Input: part model. Units: mm. Frame: model coordinates. A direction names the side the tool comes from. Round coordinates to 2 decimals unless told otherwise and drop trailing zeros. Loops run counter-clockwise (first coordinate to the right, second up) from the corner with the lowest first, then second, coordinate; pieces in that order, holes last. Notation, with made-up numbers: M 35.5,-40 L 57.5,-40 A22 cw 57.5,-2 Z; hole C -0.75,18.25 d2. An arc over 180 degrees is marked long. Return JSON: item names as keys, results as strings. Group by question number.
1) Contact query for flat-ended pins moving along their axis: P1, Ø1.2, axis at x = -194.5, z = 1.5, coming from the +Y side; P2, Ø1.5, axis at y = 70.5, z = 0.5, coming from the -X side. Output: stop coordinate, or through.
2) Mould query, pull axis X, two halves, no side actions, for faces 3 (the face through (-199.298, 76, 1)), 4 (the face through (-157, 69.019, 1)), 5 (the face through (-119.098, 79, 1)), 6 (the face through (-113.953, 82.117, 1.234)). Classes: +X half, -X half, draft (parallel to the pull), parting line (faces both ways), or undercut.
3) Access query for faces 1 (the face through (-113.098, 76, 1)), 2 (the face through (-118, 76.019, 1)). Directions: +Z, -Z, +X, -X, +Y, -Y. A direction counts if a zero-diameter tool reaches every point of the face in a straight line with its end or side. Return the directions, or none.
4) Section B-B (z = 0.95). Output: boundary loops of the cut face in (x, y), plus the area to 3 significant figures.
5) Material intervals for line 1 (X direction, y = 78.75, z = 0.55); line 2 (X direction, y = 72.25, z = 0.2); line 3 (X direction, y = 70.75, z = 1.6), sorted ascending. Write a range as from..to.
6) Section A-A (y = 78.5). Output: boundary loops of the cut face in (x, z).
from build123d import *

# Parameters (mm, degrees)
RESSALTO_EXTRUS_O1_DEPTH = 2.5
FILETE1_R                = 0.1


with BuildPart() as part:
    # Esboço1 → Ressalto-extrusão1 (new body)
    with BuildSketch(Plane.XY):
        with BuildLine():
            ThreePointArc((-199.297641475, 72.518779678), (-198.272493356, 70.044033295), (-195.797641475, 69.019139891))
            Line((-195.797641475, 69.019139891), (-116.597641475, 69.019139891))
            ThreePointArc((-116.597641475, 69.019139891), (-114.122789593, 70.044033295), (-113.097641475, 72.518779678))
            Line((-113.097641475, 72.518779678), (-113.097641475, 80.019139873))
            ThreePointArc((-113.097641475, 80.019139873), (-113.976321131, 82.140460216), (-116.097641475, 83.019139873))
            Line((-116.097641475, 83.019139873), (-116.597641475, 83.019139873))
            Line((-116.597641475, 83.019139873), (-116.597641475, 76.019139873))
            Line((-116.597641475, 76.019139873), (-119.097641475, 76.019139873))
            Line((-119.097641475, 76.019139873), (-119.097641475, 83.019139873))
            Line((-119.097641475, 83.019139873), (-135.097641475, 83.019139873))
            Line((-135.097641475, 83.019139873), (-141.097641475, 83.019139873))
            Line((-141.097641475, 83.019139873), (-171.297641475, 83.019139873))
            Line((-171.297641475, 83.019139873), (-177.297641475, 83.019139873))
            Line((-177.297641475, 83.019139873), (-193.297641475, 83.019139873))
            Line((-193.297641475, 83.019139873), (-193.297641475, 76.019139873))
            Line((-193.297641475, 76.019139873), (-195.797641475, 76.019139873))
            Line((-195.797641475, 76.019139873), (-195.797641475, 83.019139873))
            Line((-195.797641475, 83.019139873), (-196.297641475, 83.019139873))
            ThreePointArc((-196.297641475, 83.019139873), (-198.418961818, 82.140460216), (-199.297641475, 80.019139873))
            Line((-199.297641475, 80.019139873), (-199.297641475, 72.518779678))
        make_face()
    extrude(amount=RESSALTO_EXTRUS_O1_DEPTH)

    # Filete1
    filete1_edges = [part.edges().sort_by_distance(p)[0] for p in [
        (-199.297641475, 76.268959775, 2.5),
        (-195.797641475, 79.519139873, 0),
        (-194.547641475, 76.019139873, 0),
        (-198.272493356, 70.044033295, 2.5),
        (-193.297641475, 79.519139873, 0),
        (-156.197641475, 83.019139873, 0),
        (-119.097641475, 79.519139873, 0),
        (-117.847641475, 76.019139873, 0),
        (-116.597641475, 79.519139873, 0),
        (-116.347641475, 83.019139873, 0),
        (-113.976321131, 82.140460216, 0),
        (-113.097641475, 76.268959775, 0),
        (-156.197641475, 69.019139891, 2.5),
        (-114.122789593, 70.044033295, 0),
        (-156.197641475, 69.019139891, 0),
        (-198.272493356, 70.044033295, 0),
        (-199.297641475, 76.268959775, 0),
        (-198.418961818, 82.140460216, 0),
        (-196.047641475, 83.019139873, 0),
        (-114.122789593, 70.044033295, 2.5),
        (-113.097641475, 76.268959775, 2.5),
        (-195.797641475, 83.019139873, 1.25),
        (-195.797641475, 76.019139873, 1.25),
        (-193.297641475, 76.019139873, 1.25),
        (-193.297641475, 83.019139873, 1.25),
        (-119.097641475, 83.019139873, 1.25),
        (-119.097641475, 76.019139873, 1.25),
        (-116.597641475, 76.019139873, 1.25),
        (-116.597641475, 83.019139873, 1.25),
        (-113.976321131, 82.140460216, 2.5),
        (-116.347641475, 83.019139873, 2.5),
        (-116.597641475, 79.519139873, 2.5),
        (-117.847641475, 76.019139873, 2.5),
        (-119.097641475, 79.519139873, 2.5),
        (-196.047641475, 83.019139873, 2.5),
        (-156.197641475, 83.019139873, 2.5),
        (-193.297641475, 79.519139873, 2.5),
        (-194.547641475, 76.019139873, 2.5),
        (-195.797641475, 79.519139873, 2.5),
        (-198.418961818, 82.140460216, 2.5),
    ]]
    fillet(filete1_edges, radius=FILETE1_R)


solid = part.part
Returned:
{
 "1": {"P1": "stops at y = 76.02", "P2": "stops at x = -199.06"},
 "2": {"face 3": "-X half", "face 4": "draft", "face 5": "undercut", "face 6": "+X half"},
 "3": {"face 1": "+Z, -Z, +X, +Y, -Y", "face 2": "+Z, -Z, +Y"},
 "4": {"outline": "M -199.3,72.52 A3.5 ccw -195.8,69.02 L -116.6,69.02 A3.5 ccw -113.1,72.52 L -113.1,80.02 A3 ccw -116.1,83.02 L -116.5,83.02 A0.1 ccw -116.6,82.92 L -116.6,76.12 A0.1 cw -116.7,76.02 L -119,76.02 A0.1 cw -119.1,76.12 L -119.1,82.92 A0.1 ccw -119.2,83.02 L -193.2,83.02 A0.1 ccw -193.3,82.92 L -193.3,76.12 A0.1 cw -193.4,76.02 L -195.7,76.02 A0.1 cw -195.8,76.12 L -195.8,82.92 A0.1 ccw -195.9,83.02 L -196.3,83.02 A3 ccw -199.3,80.02 Z", "area": "1,160 mm^2"},
 "5": {"line 1": "x = -199.3..-195.8, -193.3..-119.1, -116.6..-113.1", "line 2": "x = -199.29..-113.11", "line 3": "x = -198.82..-113.58"},
 "6": {"outline": "M -199.3,0.1 A0.1 ccw -199.2,0 L -195.9,0 A0.1 ccw -195.8,0.1 L -195.8,2.4 A0.1 ccw -195.9,2.5 L -199.2,2.5 A0.1 ccw -199.3,2.4 Z; M -193.3,0.1 A0.1 ccw -193.2,0 L -119.2,0 A0.1 ccw -119.1,0.1 L -119.1,2.4 A0.1 ccw -119.2,2.5 L -193.2,2.5 A0.1 ccw -193.3,2.4 Z; M -116.6,0.1 A0.1 ccw -116.5,0 L -113.2,0 A0.1 ccw -113.1,0.1 L -113.1,2.4 A0.1 ccw -113.2,2.5 L -116.5,2.5 A0.1 ccw -116.6,2.4 Z"}
}
